```python
from build123d import *

# Parameters (mm, degrees)
CROQUIS1_R              = 155
CROQUIS1_R_2            = 33.0759403
SALIENTE_EXTRUIR1_DEPTH = 10
CROQUIS3_R              = 159.665159843
CROQUIS3_R_2            = 147.665159843
SALIENTE_EXTRUIR2_DEPTH = 12.5


with BuildPart() as part:
    # Croquis1 → Saliente-Extruir1 (new, symmetric)
    with BuildSketch(Plane(origin=(0, 0, 0), x_dir=(1, 0, 0), z_dir=(0, 1, 0))):
        with Locations(Location((0, 0, 0), (0, 0, 270))):
            Circle(CROQUIS1_R)
        with Locations(Location((0, 95.059598075, 0), (0, 0, 270))):
            Circle(CROQUIS1_R_2, mode=Mode.SUBTRACT)
        with Locations(Location((82.324026806, 47.529799037, 0), (0, 0, 270))):
            Circle(CROQUIS1_R_2, mode=Mode.SUBTRACT)
        with Locations(Location((82.324026806, -47.529799037, 0), (0, 0, 270))):
            Circle(CROQUIS1_R_2, mode=Mode.SUBTRACT)
        with Locations(Location((0, -95.059598075, 0), (0, 0, 270))):
            Circle(CROQUIS1_R_2, mode=Mode.SUBTRACT)
        with Locations(Location((-82.324026806, -47.529799037, 0), (0, 0, 270))):
            Circle(CROQUIS1_R_2, mode=Mode.SUBTRACT)
        with Locations(Location((-82.324026806, 47.529799037, 0), (0, 0, 270))):
            Circle(CROQUIS1_R_2, mode=Mode.SUBTRACT)
        with BuildLine():
            Line((-2, 16.5), (2, 16.5))
            Line((2, 16.5), (2, 14.866068747))
            ThreePointArc((2, 14.866068747), (0, -15), (-2, 14.866068747))
            Line((-2, 14.866068747), (-2, 16.5))
        make_face(mode=Mode.SUBTRACT)
    extrude(amount=SALIENTE_EXTRUIR1_DEPTH, both=True)

    # Croquis2 → Revolución1 (revolve)
    with BuildSketch(Plane(origin=(0, 0, 0), x_dir=(0, 0, -1), z_dir=(1, 0, 0)), mode=Mode.PRIVATE) as revoluci_n1_sk:
        Polygon((155, 10), (155, 4.5), (159.641767411, 7), (159.641767411, 10), align=None)
        Polygon((155, -4.5), (155, -10), (159.641767411, -10), (159.641767411, -7), align=None)
    revolve(revoluci_n1_sk.sketch.rotate(Axis((0, 10, 0), (0, -1, 0)), 180), axis=Axis((0, 10, 0), (0, -1, 0)))

    # Croquis3 → Saliente-Extruir2 (add)
    with BuildSketch(Plane(origin=(0, 10, 0), x_dir=(1, 0, 0), z_dir=(0, 1, 0))):
        with Locations(Location((0, 0, 0), (0, 0, 270))):
            Circle(CROQUIS3_R)
        with Locations(Location((0, 0, 0), (0, 0, 270))):
            Circle(CROQUIS3_R_2, mode=Mode.SUBTRACT)
    saliente_extruir2 = extrude(amount=SALIENTE_EXTRUIR2_DEPTH)

    # Simetría1: Saliente-Extruir2 across plane
    add(saliente_extruir2.mirror(Plane.ZX))


solid = part.part
```
The listing builds one solid part. Answer for the finished solid, in the listing's coordinates (mm). A direction names the side the tool comes from. Round coordinates to 2 decimals unless told otherwise and drop trailing zeros. Loops run counter-clockwise (first coordinate to the right, second up) from the corner with the lowest first, then second, coordinate; pieces in that order, holes last. Notation, with made-up numbers: (-19.75, 80.5) - (39.25, 80.5) arc R15 ccw to (39.25, 91.5) - close; hole circle Ø3 at (62, 39). An arc over 180 degrees is marked (long way). Return JSON: item names as keys, results as strings. Group by question number.
1. Which of the six approach directions +Z, -Z, +X, -X, +Y, -Y give full straight-line access (tool end or side, diameter ignored) to faces 5 (the flat face through (-2, -10, -31)), 6 (the conical face through (-153.9, -4.62, -20.21)), 7 (the cylindrical face through (-47.95, 8.52, 152.27)), 8 (the cylindrical face through (44.355, 16.163, 140.846)), 9 (the flat face through (-47, 22.5, 141))?
2. The mould has two halves that part along Z. Classify faces 1 (the flat face through (-47, -22.5, 141)), 2 (the cylindrical face through (-54.434, -0.14, 65.311)), 3 (the cylindrical face through (-59.37, 0.06, 143.18)), 4 (the cylindrical face through (69.7, -0.1, 78.1)): pulls with the +Z half, pulls with the -Z half, needs draft (parallel to the pull), parting line crosses it, or undercut.
3. The part is cut by section B-B on y = -18. Determine the outline of the cut face in (x, z), then the cut area to 3 significant figures.
4. Each of these flat-tipped pins is pushed along its axis until it touches: P1, Ø4, axis at x = -113.5, z = -20.5, coming from the +Y side; P2, Ø3, axis at x = -118, z = -62, coming from the -Y side; P3, Ø8, axis at y = -5, z = -122, coming from the -X side; P4, Ø24, axis at x = 0, z = 0, coming from the +Y side. Where does it stop, or does it pass through?
5. Consider probe 1 along Z at (x, y) = (1, 18); probe 2 along X at (y, z) = (9.5, -33); probe 3 along Z at (x, y) = (-20.5, 6). Determine where each line is inside the solid, lowest interval first.
6. The part is cut by section C-C on x = 96. State how many separate pieces and enclosed holes the cut face has, then the cut area to 3 significant figures.
Resolved:
{
 "1": {"face 5": "-Y", "face 6": "none", "face 7": "+Y, -Y", "face 8": "+Y", "face 9": "+Z, -Z, +X, -X, +Y"},
 "2": {"face 1": "needs draft", "face 2": "undercut", "face 3": "parting line crosses it", "face 4": "undercut"},
 "3": {"outline": "circle Ø319.33 at (0, 0); hole circle Ø295.33 at (0, 0)", "area": "11,600 mm²"},
 "4": {"P1": "stops at y = 10", "P2": "stops at y = -10", "P3": "stops at x = -106.93", "P4": "passes through"},
 "5": {"probe 1": "z = -159.66 to -147.66, 147.66 to 159.66", "probe 2": "x = -156.19 to -112.04, -52.61 to 52.61, 112.04 to 156.19", "probe 3": "z = -156.45 to -121.02, -69.1 to 69.1, 121.02 to 156.45"},
 "6": {"separate pieces": "3", "enclosed holes": "0", "area": "3,330 mm²"}
}
